The figure shows three views and two pictorial views of one solid part (mm, origin at its lowest corner). Answer the questions. A direction names the side the tool comes from. Give positions to 0.01 mm unless a question says otherwise; leave off trailing zeros. Write each loop counter-clockwise with the first axis right and the second up, starting at its lowest first coordinate (ties: lowest second). Pieces come first, ordered by that corner, then holes. Notation, with made-up numbers: (-10, 8) -> (49, 8) arc R17 cw to (49, 23) -> close; hole circle Ø3 at (-34.5, -0.5). An arc over 180 degrees is marked (long way). Use a Markdown table: item, result.
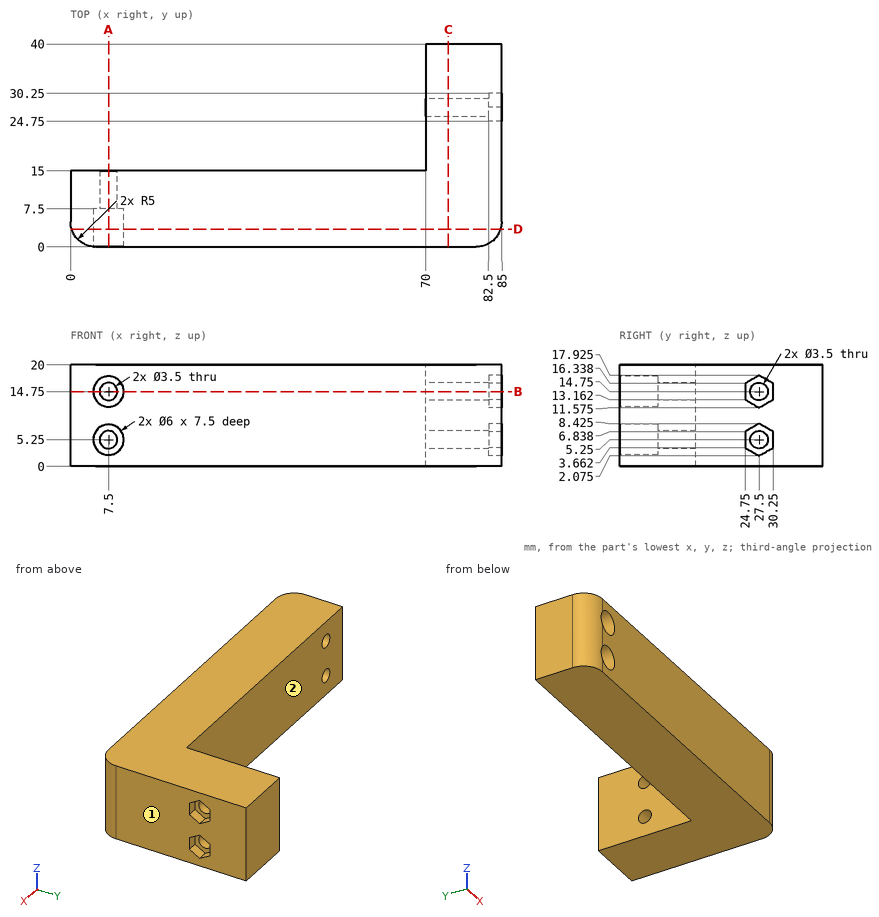
Item 1: Each of these flat-tipped pins is pushed along its axis until it touches: P1, Ø3, axis at x = 7.5, z = 5.25, coming from the -Y side; P2, Ø2, axis at x = 83, z = 15, coming from the -Y side; P3, Ø6, axis at y = 31.5, z = 12, coming from the -X side; P4, Ø4.5, axis at y = 26, z = 4, coming from the +X side. Where does it stop, or does it pass through?
Return value:
| item | result |
|---|---|
| P1 | through |
| P2 | y = 0.42 |
| P3 | x = 70 |
| P4 | x = 85 |
Item 2: A cutting plane is placed at D-D (y = 3.5). Give the vertices of the cut face in (x, z).
Return value:
| item | result |
|---|---|
| outline | (0.23, 0) -> (84.77, 0) -> (84.77, 20) -> (0.23, 20) -> close; hole circle Ø6 at (7.5, 5.25); hole circle Ø6 at (7.5, 14.75) |
Item 3: Straight lines are drawn through the part: line 1 along Z through (x, y) = (7.5, 10); line 2 along Z through (x, y) = (7, 5); line 3 along Y through (x, z) = (45, 3.5). For each, find the intervals that lie inside material, in ascending order. Write a range as [from, to].
Return value:
| item | result |
|---|---|
| line 1 | [0, 3.5], [7, 13], [16.5, 20] |
| line 2 | [0, 2.29], [8.21, 11.79], [17.71, 20] |
| line 3 | [0, 15] |
Item 4: A cutting plane is placed at A-A (x = 7.5). Give the vertices of the cut face in (y, z).
Return value:
| item | result |
|---|---|
| outline | (0, 0) -> (15, 0) -> (15, 3.5) -> (7.5, 3.5) -> (7.5, 2.25) -> (0, 2.25) -> close; (0, 8.25) -> (7.5, 8.25) -> (7.5, 7) -> (15, 7) -> (15, 13) -> (7.5, 13) -> (7.5, 11.75) -> (0, 11.75) -> close; (0, 17.75) -> (7.5, 17.75) -> (7.5, 16.5) -> (15, 16.5) -> (15, 20) -> (0, 20) -> close |
Item 5: A cutting plane is placed at B-B (z = 14.75). Count the separate pieces of the cut face and the enclosed holes in it, then the cut area to 3 significant figures.
Return value:
| item | result |
|---|---|
| separate pieces | 3 |
| enclosed holes | 0 |
| area | 1,510 mm^2 |
Item 6: A cutting plane is placed at C-C (x = 74.5). Give the vertices of the cut face in (y, z), then the cut area to 3 significant figures.
Return value:
| item | result |
|---|---|
| outline | (0, 0) -> (40, 0) -> (40, 20) -> (0, 20) -> close; hole circle Ø3.5 at (27.5, 5.25); hole circle Ø3.5 at (27.5, 14.75) |
| area | 781 mm^2 |
Item 7: A tool of negligible diameter and unlimited length cuts with its end or side. For the marked faces 1 and 2, from which of +Z, -Z, +X, -X, +Y, -Y can it reach the whole face along a straight path? Write none if from no direction.
Return value:
| item | result |
|---|---|
| face 1 | +Z, -Z, +X, +Y, -Y |
| face 2 | +Z, -Z, -X, +Y |
